Check sheet for the drawn part. Datum: minimum x, y, z corner. Units: mm. A direction names the side the tool comes from. Coordinates: 2 decimals unless noted, no trailing zeros. Write each loop counter-clockwise with the first axis right and the second up, starting at its lowest first coordinate (ties: lowest second). Pieces come first, ordered by that corner, then holes. Notation, with made-up numbers: M 64.25,88 L 75.25,88 A21 ccw 75.25,122 Z; hole C 23,-28.75 d6. An arc over 180 degrees is marked long. Answer as CSV lines item,"result". Start each with the question number.
Q1. Sectioned sample at D-D, the plane x = 19. Record the cut outline in (y, z), then the cut area to 3 significant figures.
Q2. Access from +Z, -Z, +X, -X, +Y, -Y to the whole of each face (thin tool, end or side, straight path). Record for the marked faces 4, 5 and 6.
Q3. Thickness scan on line 1 along X through (y, z) = (21.25, 30.5) (1 decimal); line 2 along Z through (x, y) = (15.5, 16); line 3 along Y through (x, z) = (11.5, 30). Record the ranges inside material, lowest first. Write a range as from..to.
Q4. Sectioned sample at A-A, the plane x = 5.08. Record the cut outline in (y, z) (1 decimal).
Q5. Sectioned sample at C-C, the plane y = 16.25. Record the cut outline in (x, z).
Q6. Sectioned sample at B-B, the plane z = 33. Record the cut outline in (x, y).
Q7. Mould release check, pull along Z, two halves, no side actions. Record for the marked faces 1, 2 and 3: pulls with the +Z half, pulls with the -Z half, needs draft (parallel to the pull), parting line crosses it, or undercut.
Q8. Depth check by flat-ended pin: pin 1 Ø1.5 at (x, y) = (20.5, 14) entering from +Z; pin 2 Ø5 at (x, z) = (20.5, 22) entering from +Y (1 decimal); pin 3 Ø4 at (x, z) = (15.24, 31.877) entering from -Y; pin 4 Ø6 at (x, z) = (3.5, 26) entering from -Y. Enter the tip coordinate at first touch or a pass-through.
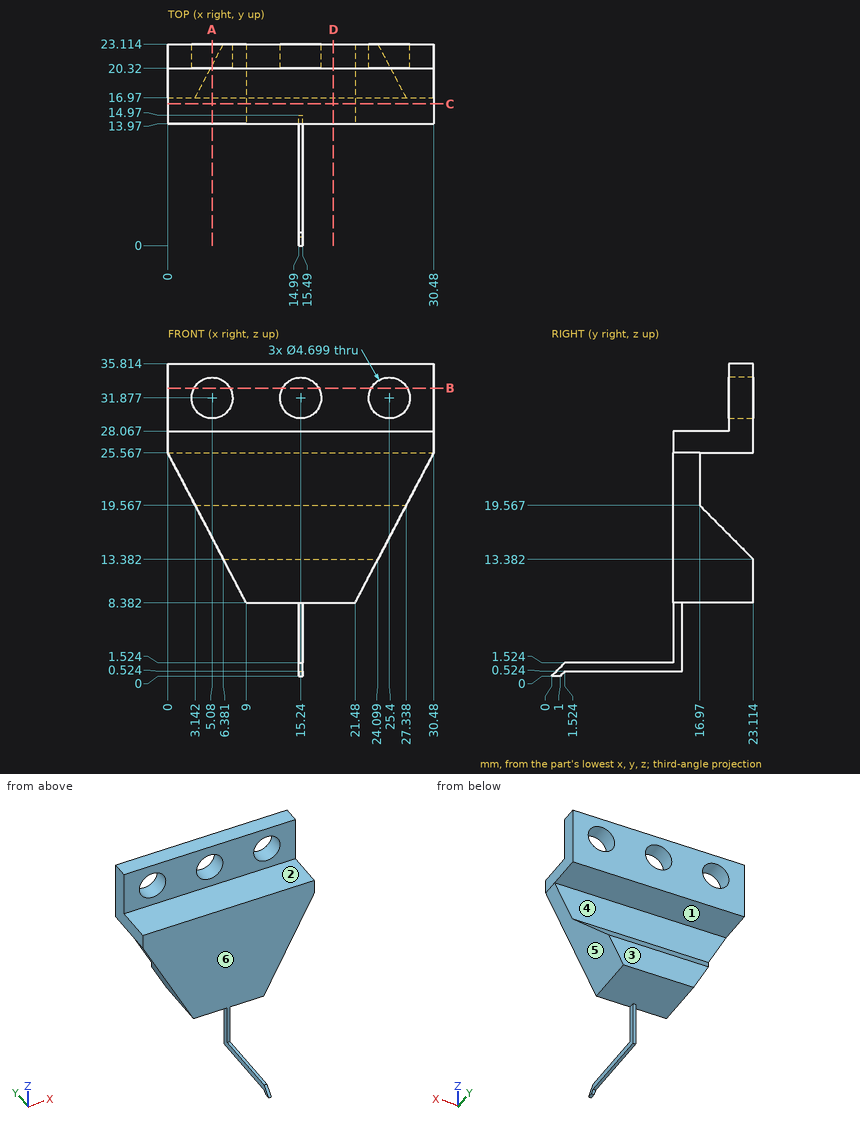
Output:
1,outline,"M 13.97,8.38 L 23.11,8.38 L 23.11,13.38 L 16.97,19.57 L 16.97,25.57 L 23.11,25.57 L 23.11,35.81 L 20.32,35.81 L 20.32,28.07 L 13.97,28.07 Z"
1,area,"146 mm^2"
2,face 4,"+X, -X, +Y"
2,face 5,"-Z, +X, +Y, -Y"
2,face 6,"+Z, +X, -X, -Y"
3,line 1,"x = 0..3.2, 7..13.3, 17.1..23.5, 27.3..30.5"
3,line 2,"z = 8.38..28.07"
3,line 3,"y = 20.32..23.11"
4,outline,"M 14,15.9 L 20.6,15.9 L 17,19.6 L 17,25.6 L 23.1,25.6 L 23.1,29.5 L 20.3,29.5 L 20.3,28.1 L 14,28.1 Z; M 20.3,34.2 L 23.1,34.2 L 23.1,35.8 L 20.3,35.8 Z"
5,outline,"M 0,25.57 L 9,8.38 L 21.48,8.38 L 30.48,25.57 L 30.48,28.07 L 0,28.07 Z"
6,outline,"M 0,20.32 L 3.02,20.32 L 3.02,23.11 L 0,23.11 Z; M 7.14,20.32 L 13.18,20.32 L 13.18,23.11 L 7.14,23.11 Z; M 17.3,20.32 L 23.34,20.32 L 23.34,23.11 L 17.3,23.11 Z; M 27.46,20.32 L 30.48,20.32 L 30.48,23.11 L 27.46,23.11 Z"
7,face 1,"undercut"
7,face 2,"pulls with the +Z half"
7,face 3,"needs draft"
8,pin 1,"stops at z = 28.07"
8,pin 2,"stops at y = 17"
8,pin 3,"passes through"
8,pin 4,"stops at y = 13.97"
